Geometry check sheet. Reference: the model listing, model coordinates, mm. Give positions to 0.01 mm unless a question says otherwise; leave off trailing zeros. Order: outer loops, then holes, each group sorted by start corner. A loop starts at its lowest first (then second) coordinate and runs counter-clockwise, first axis right, second up.
from build123d import *

# Parameters (mm, degrees)
PAD_DEPTH   = 3
FILLET_R    = 1
FILLET001_R = 1


with BuildPart() as part:
    # Sketch → Pad (new body)
    with BuildSketch(Plane.XY):
        Polygon((-3.25, 0), (3.25, 0), (1, 7), (-1, 7), align=None)
    extrude(amount=PAD_DEPTH)

    # Fillet
    fillet_edges = [part.edges().sort_by_distance(p)[0] for p in [
        (-3.25, 0, 1.5),
        (3.25, 0, 1.5),
        (1, 7, 1.5),
        (-1, 7, 1.5),
    ]]
    fillet(fillet_edges, radius=FILLET_R)

    # Fillet001
    fillet001_edges = [part.edges().sort_by_distance(p)[0] for p in [
        (0, 0, 3),
        (-2.68627, 0.410937, 3),
        (2.68627, 0.410937, 3),
        (-2.02664, 3.806009, 3),
        (2.02664, 3.806009, 3),
        (-0.860103, 6.808087, 3),
        (0.860103, 6.808087, 3),
        (0, 7, 3),
    ]]
    fillet(fillet001_edges, radius=FILLET001_R)


solid = part.part
Item 1: Sectioned sample at B-B (z = 0.5). Enter the section's corners in (x, y).
Reported:
outline: (-2.83, 1.31) arc R1 ccw to (-1.88, 0) - (1.88, 0) arc R1 ccw to (2.83, 1.31) - (1.22, 6.31) arc R1 ccw to (0.27, 7) - (-0.27, 7) arc R1 ccw to (-1.22, 6.31) - close
Item 2: Sectioned sample at A-A (z = 2.65). Enter the section's corners in (x, y).
Reported:
outline: (-2.6, 1.23) arc R0.76 ccw to (-1.88, 0.24) - (1.88, 0.24) arc R0.76 ccw to (2.6, 1.23) - (0.99, 6.23) arc R0.76 ccw to (0.27, 6.76) - (-0.27, 6.76) arc R0.76 ccw to (-0.99, 6.23) - close
Item 3: Gauge pin test, flat end, axial feed: pin 1 (1 mm diameter, centred on y = 5.5, z = 1.5, fed in from +X). Record the tip position at first contact, or that the pin passes through.
Reported:
pin 1: stops at x = 1.64
Item 4: Draft check along X on faces 1 (the cylindrical face through (-0.853, 6.813, 1.014)), 2 (the flat face through (2.04, 3.77, 0.99)), 3 (the flat face through (0, 3, 0)). Enter one of: released by +X, released by -X, zero draft, split by the parting line, or undercut.
Reported:
face 1: released by -X
face 2: released by +X
face 3: zero draft
Item 5: Scan lines: L1, parallel to Y at x = 0.7, z = 2.65; L2, parallel to X at y = 4.25, z = 0.3; L3, parallel to X at y = 6, z = 0.6. Record each from-to range of solid material in increasing order.
Reported:
L1: y = 0.24 to 6.63
L2: x = -1.88 to 1.88
L3: x = -1.32 to 1.32
